from build123d import *

# Parameters (mm, degrees)
SKETCH_1_W          = 55
SKETCH_1_H          = 30
SKETCH_1_R          = 11
EXTRUDE_1_DEPTH     = 15
SKETCH_2_R          = 2.55
CUT_EXTRUDE_1_DEPTH = 44.373378932
SKETCH_4_R          = 12
CUT_EXTRUDE_3_DEPTH = 1
CUT_EXTRUDE_START   = -1
SKETCH_5_R          = 12
CUT_EXTRUDE_4_DEPTH = 1
SKETCH_6_R          = 1.2
CUT_EXTRUDE_5_DEPTH = 35.731109974
FILLET_2_R          = 1
SKETCH_7_R          = 4.5
CUT_EXTRUDE_6_DEPTH = 6


with BuildPart() as part:
    # 草图1 → 凸台-拉伸1 (new body)
    with BuildSketch(Plane.XY):
        Rectangle(SKETCH_1_W, SKETCH_1_H)
        Circle(SKETCH_1_R, mode=Mode.SUBTRACT)
    extrude(amount=EXTRUDE_1_DEPTH)

    # 草图2 → 切除-拉伸1 (cut, through all)
    with BuildSketch(Plane(origin=(0, 15, 0), x_dir=(1, 0, 0), z_dir=(0, 1, 0))):
        with Locations(Location((-20, -7.5, 0), (0, 0, 270))):
            Circle(SKETCH_2_R)
        with Locations(Location((20, -7.5, 0), (0, 0, 90))):
            Circle(SKETCH_2_R)
    extrude(amount=-CUT_EXTRUDE_1_DEPTH, mode=Mode.SUBTRACT)

    # 草图4 → 切除-拉伸3 (cut)
    with BuildSketch(Plane(origin=(0, 0, 0), x_dir=(-1, 0, 0), z_dir=(0, 0, -1))):
        Circle(SKETCH_4_R)
    extrude(amount=-CUT_EXTRUDE_3_DEPTH, mode=Mode.SUBTRACT)

    # 草图5 → 切除-拉伸4 (cut)
    with BuildSketch(Plane.XY.offset(15).offset(CUT_EXTRUDE_START)):
        with Locations(Location((0, 0, 0), (0, 0, 180))):
            Circle(SKETCH_5_R)
    extrude(amount=CUT_EXTRUDE_4_DEPTH, mode=Mode.SUBTRACT)

    # 草图6 → 切除-拉伸5 (cut, through all)
    with BuildSketch(Plane.XY.offset(15)):
        with Locations((12, 12)):
            Circle(SKETCH_6_R)
        with Locations(Location((-12, 12, 0), (0, 0, 180))):
            Circle(SKETCH_6_R)
        with Locations((-12, -12)):
            Circle(SKETCH_6_R)
        with Locations(Location((12, -12, 0), (0, 0, 180))):
            Circle(SKETCH_6_R)
    extrude(amount=-CUT_EXTRUDE_5_DEPTH, mode=Mode.SUBTRACT)

    # 圆角2
    fillet_2_edges = [part.edges().sort_by_distance(p)[0] for p in [
        (-27.5, 15, 7.5),
        (27.5, 15, 7.5),
        (27.5, -15, 7.5),
        (-27.5, -15, 7.5),
    ]]
    fillet(fillet_2_edges, radius=FILLET_2_R)

    # 草图7 → 切除-拉伸6 (cut)
    with BuildSketch(Plane(origin=(0, 15, 0), x_dir=(1, 0, 0), z_dir=(0, 1, 0))):
        with Locations(Location((-20, -7.5, 0), (0, 0, 270))):
            Circle(SKETCH_7_R)
        with Locations(Location((20, -7.5, 0), (0, 0, 270))):
            Circle(SKETCH_7_R)
    extrude(amount=-CUT_EXTRUDE_6_DEPTH, mode=Mode.SUBTRACT)


solid = part.part
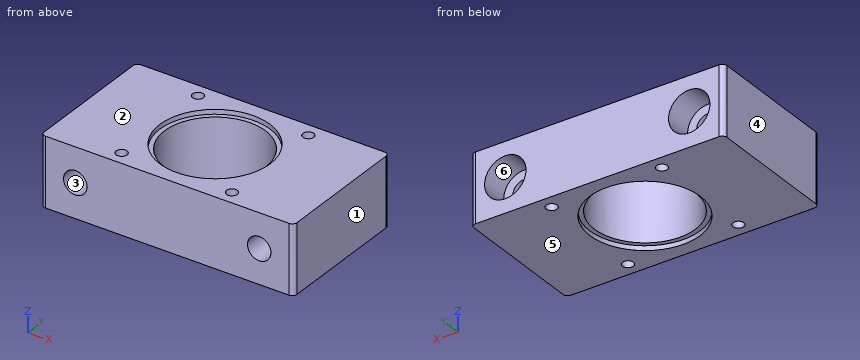
CAD build for the part. Positions are in the model's coordinates, mm. Face numbers are marked on the shaded views. A direction names the side the tool comes from. Round coordinates to 2 decimals unless told otherwise and drop trailing zeros. Order: outer loops, then holes, each group sorted by start corner. A loop starts at its lowest first (then second) coordinate and runs counter-clockwise, first axis right, second up. Notation, with made-up numbers: (-8.5, -24.75) - (-0.5, -24.75) arc R19 cw to (-0.5, -9.75) - close; hole circle Ø6 at (50, 69). An arc over 180 degrees is marked (long way). Return JSON: item names as keys, results as strings.
(1) Pin check, flat tips, straight feed: pin 1 Ø12 at (x, y) = (-1, 4.5) entering from -Z; pin 2 Ø8 at (x, z) = (-20, 7.5) entering from +Y. Stop position of each tip, or through.
Answer key:
{"pin 1": "passes through", "pin 2": "stops at y = 9"}
(2) Cut at A-A (z = 7.5). State how many separate pieces and enclosed holes the cut face has, then the cut area to 3 significant figures.
Answer key:
{"separate pieces": "3", "enclosed holes": "5", "area": "898 mm^2"}
(3) Cut at B-B (y = 6). Give the cut face in (x, z).
Answer key:
{"outline": "(-27.5, 0) - (-10.39, 0) - (-10.39, 1) - (-9.22, 1) - (-9.22, 14) - (-10.39, 14) - (-10.39, 15) - (-27.5, 15) - close; (9.22, 1) - (10.39, 1) - (10.39, 0) - (27.5, 0) - (27.5, 15) - (10.39, 15) - (10.39, 14) - (9.22, 14) - close; hole circle Ø5.1 at (-20, 7.5); hole circle Ø5.1 at (20, 7.5)"}
(4) Wall check: probe 1 along Y at (x, z) = (-12, 8); probe 2 along Y at (x, z) = (-0.5, 3.75); probe 3 along Z at (x, y) = (20, -6). Give the ranges that are in metal, low to high. Write a range as from..to.
Answer key:
{"probe 1": "y = -15..-13.2, -10.8..10.8, 13.2..15", "probe 2": "y = -15..-10.99, 10.99..15", "probe 3": "z = 0..4.95, 10.05..15"}
(5) Cut at C-C (x = -20). Give the cut face in (y, z), then the cut area to 3 significant figures.
Answer key:
{"outline": "(-15, 0) - (15, 0) - (15, 3) - (9, 3) - (9, 4.95) - (-15, 4.95) - close; (-15, 10.05) - (9, 10.05) - (9, 12) - (15, 12) - (15, 15) - (-15, 15) - close", "area": "274 mm^2"}
(6) Tool access for the marked faces 5 and 6: list every direction of +Z, -Z, +X, -X, +Y, -Y with a clear straight run to the whole face (end or side of a thin tool).
Answer key:
{"face 5": "-Z, +X, -X, +Y, -Y", "face 6": "+Y"}
(7) Pull direction X, two halves, no side cores. Call the marked faces 1, 2, 3 and 4: +X half, -X half, draft (parallel to the pull), parting line (faces both ways), or undercut.
Answer key:
{"face 1": "+X half", "face 2": "draft", "face 3": "undercut", "face 4": "-X half"}
(8) Cut at D-D (y = -9). Give the cut face in (x, z).
Answer key:
{"outline": "(-27.5, 0) - (-7.94, 0) - (-7.94, 1) - (-6.32, 1) - (-6.32, 14) - (-7.94, 14) - (-7.94, 15) - (-27.5, 15) - close; (6.32, 1) - (7.94, 1) - (7.94, 0) - (27.5, 0) - (27.5, 15) - (7.94, 15) - (7.94, 14) - (6.32, 14) - close; hole circle Ø5.1 at (-20, 7.5); hole circle Ø5.1 at (20, 7.5)"}
